Geometry check sheet. Reference: the model listing, model coordinates, mm. A direction names the side the tool comes from. Round coordinates to 2 decimals unless told otherwise and drop trailing zeros. Write each loop counter-clockwise with the first axis right and the second up, starting at its lowest first coordinate (ties: lowest second). Pieces come first, ordered by that corner, then holes. Notation, with made-up numbers: M 36.5,10 L 74.5,10 A13 ccw 74.5,21 Z; hole C 64,0 d11. An arc over 180 degrees is marked long. Put each result on its own line as item: value. Start each with the question number.
(1) Material ranges on probe 1 along X at (y, z) = (13.75, -4.5) (3 decimals); probe 2 along X at (y, z) = (8, -6.5) (3 decimals); probe 3 along X at (y, z) = (10.5, -2.75), recorded low to high.
(2) Section check A-A on y = 12.25. Record the cut outline in (x, z) (3 decimals).
(3) Section check B-B on y = 17.25. Record the cut outline in (x, z).
(4) Mould release check, pull along Y, two halves, no side actions. Record for faces 1 (the flat face through (-1.6, 1, 0)), 2 (the cylindrical face through (-3.24, 4.33, 3.54)), 3 (the flat face through (0, 1.5, -2)): pulls with the +Y half, pulls with the -Y half, needs draft (parallel to the pull), parting line crosses it, or undercut.
(5) Tool access check on faces 4 (the cylindrical face through (1.529, 0.296, 1.668)), 5 (the flat face through (1.275, 8, -6)), 6 (the flat face through (0, 1, 5)), 7 (the flat face through (2, 8, 5.4)). Record the directions out of +Z, -Z, +X, -X, +Y, -Y that give a thin tool (end or side, any length) a straight path to the whole face; none if there is none.
(6) Gauge pin test, flat ends, axial feed: pin 1 (1.8 mm diameter, centred on x = 2, y = 8.5, fed in from +Z); pin 2 (1.3 mm diameter, centred on y = 8.5, z = -6, fed in from -X) (3 decimals); pin 3 (6 mm diameter, centred on y = 8, z = 6.5, fed in from -X); pin 4 (10 mm diameter, centred on x = 5.5, z = 5.5, fed in from -Y). Record the tip position at first contact, or that the pin passes through.
from build123d import *

# Parameters (mm, degrees)
SKETCH2_W                       = 6.35
SKETCH2_H                       = 14.4
CUT_EXTRUDE1_DEPTH              = 6.2
CIRPATTERN1_COUNT               = 4
SKETCH3_W                       = 3.2
SKETCH3_H                       = 3.2
CUT_EXTRUDE2_DEPTH              = 22.644860822
SKETCH4_W                       = 1.8
SKETCH4_H                       = 1.8
CUT_EXTRUDE3_DEPTH              = 16.9608897
FILLET1_R                       = 0.5
CIRPATTERN2_COUNT               = 4
FILLET1_OF_CIRPATTERN2_R        = 0.5
SKETCH5_R                       = 0.95
CUT_EXTRUDE4_DEPTH              = 6
REVOLVE2_ANGLE                  = 90
BOSS_EXTRUDE1_DEPTH             = 1
BOSS_EXTRUDE1_DIRECTION_2_REACH = 22.576
SKETCH8_R                       = 2.2627417
CUT_EXTRUDE5_DEPTH              = 0.6


with BuildPart() as part:
    # Sketch1 → Revolve1 (revolve)
    with BuildSketch(Plane.XY, mode=Mode.PRIVATE) as revolve1_sk:
        Polygon((0, 0), (4.8, 0), (4.8, 7), (8.5, 8.8), (8.5, 19.5), (7.8, 19.5), (7.8, 15.2), (4.25, 15.2), (4.25, 9), (4, 9), (4, 1.5), (0, 1.5), align=None)
    revolve(revolve1_sk.sketch.rotate(Axis((0, 0, 0), (0, 1, 0)), 90), axis=Axis((0, 0, 0), (0, 1, 0)))

    # Sketch2 → Cut-Extrude1 (cut)
    with BuildSketch(Plane(origin=(0, 15.2, 0), x_dir=(1, 0, 0), z_dir=(0, 1, 0))):
        Rectangle(SKETCH2_W, SKETCH2_H)
    cut_extrude1 = extrude(amount=-CUT_EXTRUDE1_DEPTH, mode=Mode.SUBTRACT)

    # CirPattern1: Cut-Extrude1 ×4 about axis
    cirpattern1_axis = Axis((0, 0, 0), (0, 1, 0))
    for i in range(1, CIRPATTERN1_COUNT):
        add(cut_extrude1.rotate(cirpattern1_axis, i * 360 / CIRPATTERN1_COUNT), mode=Mode.SUBTRACT)

    # Sketch3 → Cut-Extrude2 (cut, through all)
    with BuildSketch(Plane(origin=(0, 1.5, 0), x_dir=(1, 0, 0), z_dir=(0, 1, 0))):
        Rectangle(SKETCH3_W, SKETCH3_H)
    extrude(amount=-CUT_EXTRUDE2_DEPTH, mode=Mode.SUBTRACT)

    # Sketch4 → Cut-Extrude3 (cut, through all)
    with BuildSketch(Plane(origin=(0, 9, 0), x_dir=(1, 0, 0), z_dir=(0, 1, 0))):
        with Locations((-2.175, 6.3)):
            Rectangle(SKETCH4_W, SKETCH4_H)
        with Locations((2.175, 6.3)):
            Rectangle(SKETCH4_W, SKETCH4_H)
    cut_extrude3 = extrude(amount=-CUT_EXTRUDE3_DEPTH, mode=Mode.SUBTRACT)

    # Fillet1
    fillet1_edges = [part.edges().sort_by_distance(p)[0] for p in [
        (3.075, 8.736820818, -7.2),
        (-3.075, 8.736820818, -7.2),
    ]]
    fillet(fillet1_edges, radius=FILLET1_R)

    # CirPattern2: Cut-Extrude3 ×4 about axis
    cirpattern2_axis = Axis((0, 0, 0), (0, 1, 0))
    for i in range(1, CIRPATTERN2_COUNT):
        add(cut_extrude3.rotate(cirpattern2_axis, i * 360 / CIRPATTERN2_COUNT), mode=Mode.SUBTRACT)

    # Fillet1 of CirPattern2
    fillet1_of_cirpattern2_edges = [part.edges().sort_by_distance(p)[0] for p in [
        (-7.2, 8.736820818, -3.075),
        (-7.2, 8.736820818, 3.075),
        (-3.075, 8.736820818, 7.2),
        (3.075, 8.736820818, 7.2),
        (7.2, 8.736820818, 3.075),
        (7.2, 8.736820818, -3.075),
    ]]
    fillet(fillet1_of_cirpattern2_edges, radius=FILLET1_OF_CIRPATTERN2_R)

    # Sketch5 → Cut-Extrude4 (cut)
    with BuildSketch(Plane(origin=(0, 15.2, 0), x_dir=(1, 0, 0), z_dir=(0, 1, 0))):
        with Locations(Location((4.772970773, 4.772970773, 0), (0, 0, 270))):
            Circle(SKETCH5_R)
        with Locations(Location((-4.772970773, -4.772970773, 0), (0, 0, 270))):
            Circle(SKETCH5_R)
    extrude(amount=-CUT_EXTRUDE4_DEPTH, mode=Mode.SUBTRACT)

    # Sketch6 → Revolve2 (revolve)
    with BuildSketch(Plane(origin=(0, 0, 0), x_dir=(0, 0, -1), z_dir=(1, 0, 0))):
        Polygon((-4.8, 2.8), (-6.4, 1.4), (-4.8, 0), align=None)
        Polygon((4.8, 2.8), (4.8, 0), (6.4, 1.4), align=None)
    revolve(axis=Axis((0, 0, 0), (0, 1, 0)), revolution_arc=REVOLVE2_ANGLE)

    # Sketch7 → Boss-Extrude1 (add)
    with BuildSketch(Plane(origin=(0, 2.8, 0), x_dir=(1, 0, 0), z_dir=(0, 1, 0))):
        Polygon((4.8, 0), (5.492598815, -0.721323008), (4.637239583, -1.239358321), align=None)
        Polygon((-4.8, 0), (-4.637239583, 1.239358321), (-5.492598815, 0.721323008), align=None)
    extrude(amount=BOSS_EXTRUDE1_DEPTH)

    # Boss-Extrude1 direction 2: up to this cone (the profile starts outside it)
    boss_extrude1_direction_2_end = Plane(origin=(0, 2.8, 0), z_dir=(0, -1, 0)).offset(-4.199999) * Cone(1.143e-06, 36.658285714, 32.075999, align=(Align.CENTER, Align.CENTER, Align.MIN), mode=Mode.PRIVATE)
    # Sketch7 → Boss-Extrude1 direction 2 (add, up to the surface)
    with BuildSketch(Plane(origin=(0, 2.8, 0), x_dir=(1, 0, 0), z_dir=(0, 1, 0)), mode=Mode.PRIVATE) as boss_extrude1_direction_2_sk1:
        Polygon((4.8, 0), (5.492598815, -0.721323008), (4.637239583, -1.239358321), align=None)
    boss_extrude1_direction_2_tool1 = extrude(boss_extrude1_direction_2_sk1.sketch, amount=-BOSS_EXTRUDE1_DIRECTION_2_REACH, mode=Mode.PRIVATE) - boss_extrude1_direction_2_end
    add(boss_extrude1_direction_2_tool1.solids().sort_by_distance((4.976613, 2.8, 0.65356))[0])
    # Sketch7 → Boss-Extrude1 direction 2 (add, up to the surface)
    with BuildSketch(Plane(origin=(0, 2.8, 0), x_dir=(1, 0, 0), z_dir=(0, 1, 0)), mode=Mode.PRIVATE) as boss_extrude1_direction_2_sk2:
        Polygon((-4.8, 0), (-4.637239583, 1.239358321), (-5.492598815, 0.721323008), align=None)
    boss_extrude1_direction_2_tool2 = extrude(boss_extrude1_direction_2_sk2.sketch, amount=-BOSS_EXTRUDE1_DIRECTION_2_REACH, mode=Mode.PRIVATE) - boss_extrude1_direction_2_end
    add(boss_extrude1_direction_2_tool2.solids().sort_by_distance((-4.976613, 2.8, -0.65356))[0])

    # Sketch8 → Cut-Extrude5 (cut)
    with BuildSketch(Plane.XZ):
        with Locations(Location((0, 0, 0), (0, 0, 270))):
            Circle(SKETCH8_R)
    extrude(amount=-CUT_EXTRUDE5_DEPTH, mode=Mode.SUBTRACT)


solid = part.part
Answers follow:
1. probe 1: x = -7.211 to -3.175, 3.175 to 3.863, 5.683 to 7.211
1. probe 2: x = -1.275 to 1.275
1. probe 3: x = -8.04 to -7.2, 7.2 to 8.04
2. outline: C 0,0 d17; hole M -7.2,-3.175 L -3.175,-3.175 L -3.175,-7.2 L 3.175,-7.2 L 3.175,-3.175 L 7.2,-3.175 L 7.2,3.175 L 3.175,3.175 L 3.175,7.2 L -3.175,7.2 L -3.175,3.175 L -7.2,3.175 Z; hole C -4.773,4.773 d1.9; hole C 4.773,-4.773 d1.9
3. outline: C 0,0 d17; hole C 0,0 d15.6
4. face 1: needs draft
4. face 2: undercut
4. face 3: pulls with the +Y half
5. face 4: -Y
5. face 5: +Y, -Y
5. face 6: +Z, -X, -Y
5. face 7: +Y
6. pin 1: stops at z = 8.42
6. pin 2: stops at x = -6.545
6. pin 3: stops at x = -7.7
6. pin 4: stops at y = 0
